Source: CAD feature listing. Evaluate the final solid. Frame: model axes, mm. Face numbers are marked on the shaded views. A direction names the side the tool comes from. Give positions to 0.01 mm unless a question says otherwise; leave off trailing zeros. Loops run counter-clockwise (first coordinate to the right, second up) from the corner with the lowest first, then second, coordinate; pieces in that order, holes last. Notation, with made-up numbers: M 55.5,8.25 L 95.5,8.25 A21 cw 95.5,43.25 Z; hole C 2,88.5 d2. An arc over 180 degrees is marked long. Write item = value, one per line.
from build123d import *

# Parameters (mm, degrees)
BOSS_EXTRUDE2_DEPTH  = 30
BOSS_EXTRUDE3_DEPTH  = 10
BOSS_EXTRUDE4_DEPTH  = 10
BOSS_EXTRUDE7_DEPTH  = 5
CUT_EXTRUDE9_DEPTH   = 10
SKETCH13_R           = 2.5
CUT_EXTRUDE10_DEPTH  = 190
SKETCH14_R           = 15
CUT_EXTRUDE12_DEPTH  = 15
CUT_EXTRUDE13_DEPTH  = 5
BOSS_EXTRUDE8_DEPTH  = 10
SKETCH17_R           = 5
CUT_EXTRUDE15_DEPTH  = 15
CUT_EXTRUDE16_DEPTH  = 5
SKETCH19_W           = 30
SKETCH19_H           = 5
BOSS_EXTRUDE9_DEPTH  = 5
SKETCH20_W           = 30
SKETCH20_H           = 5
BOSS_EXTRUDE10_DEPTH = 5


with BuildPart() as part:
    # Sketch2 → Boss-Extrude2 (new body)
    with BuildSketch(Plane.XY):
        Polygon((-70, 40), (-65, 45), (-5, 45), (0, 40), (0, 0), (-5, -5), (-65, -5), (-70, 0), align=None)
    extrude(amount=BOSS_EXTRUDE2_DEPTH)

    # Sketch4 → Boss-Extrude3 (add)
    with BuildSketch(Plane.XY.offset(30)):
        Polygon((-50, 45), (-45, 50), (-25, 50), (-20, 45), align=None)
    extrude(amount=-BOSS_EXTRUDE3_DEPTH)

    # Sketch5 → Boss-Extrude4 (add)
    with BuildSketch(Plane(origin=(0, 0, 0), x_dir=(-1, 0, 0), z_dir=(0, 0, -1))):
        Polygon((20, 45), (25, 50), (45, 50), (50, 45), align=None)
    extrude(amount=-BOSS_EXTRUDE4_DEPTH)

    # Sketch6 → Boss-Extrude7 (add)
    with BuildSketch(Plane.XY.offset(30)):
        Polygon((-75, 30), (5, 30), (5, 35), (-10, 35), (-10, 45), (-60, 45), (-60, 35), (-75, 35), align=None)
        Polygon((-75, 10), (5, 10), (5, 5), (-10, 5), (-10, -5), (-60, -5), (-60, 5), (-75, 5), align=None)
    extrude(amount=BOSS_EXTRUDE7_DEPTH)

    # Sketch12 → Cut-Extrude9 (cut)
    with BuildSketch(Plane.XY.offset(30)):
        with BuildLine():
            Line((-70, 25), (-60, 25))
            ThreePointArc((-60, 25), (-55, 20), (-60, 15))
            Line((-60, 15), (-70, 15))
            Line((-70, 15), (-70, 25))
        make_face()
        with BuildLine():
            Line((0, 15), (-10, 15))
            ThreePointArc((-10, 15), (-15, 20), (-10, 25))
            Line((-10, 25), (0, 25))
            Line((0, 25), (0, 15))
        make_face()
    extrude(amount=-CUT_EXTRUDE9_DEPTH, mode=Mode.SUBTRACT)

    # Sketch13 → Cut-Extrude10 (cut)
    with BuildSketch(Plane.XY.offset(20)):
        with Locations((-60, 20)):
            Circle(SKETCH13_R)
        with Locations((-10, 20)):
            Circle(SKETCH13_R)
    extrude(amount=-CUT_EXTRUDE10_DEPTH, mode=Mode.SUBTRACT)

    # Sketch14 → Cut-Extrude12 (cut)
    with BuildSketch(Plane.XY.offset(30)):
        with Locations((-35, 20)):
            Circle(SKETCH14_R)
    extrude(amount=-CUT_EXTRUDE12_DEPTH, mode=Mode.SUBTRACT)

    # Sketch15 → Cut-Extrude13 (cut)
    with BuildSketch(Plane.XY.offset(35)):
        with BuildLine():
            Line((-46.180339887, 10), (-23.819660113, 10))
            ThreePointArc((-23.819660113, 10), (-35, 5), (-46.180339887, 10))
        make_face()
        with BuildLine():
            Line((-46.180339887, 30), (-23.819660113, 30))
            ThreePointArc((-23.819660113, 30), (-35, 35), (-46.180339887, 30))
        make_face()
    extrude(amount=-CUT_EXTRUDE13_DEPTH, mode=Mode.SUBTRACT)

    # Sketch16 → Boss-Extrude8 (add)
    with BuildSketch(Plane.XY.offset(35)):
        with BuildLine():
            ThreePointArc((-17.679491924, 10), (-35, 0), (-52.320508076, 10))
            Line((-52.320508076, 10), (-46.180339887, 10))
            ThreePointArc((-46.180339887, 10), (-35, 5), (-23.819660113, 10))
            Line((-23.819660113, 10), (-17.679491924, 10))
        make_face()
        with BuildLine():
            Line((-52.320508076, 30), (-46.180339887, 30))
            ThreePointArc((-46.180339887, 30), (-35, 35), (-23.819660113, 30))
            Line((-23.819660113, 30), (-17.679491924, 30))
            ThreePointArc((-17.679491924, 30), (-35, 40), (-52.320508076, 30))
        make_face()
    extrude(amount=BOSS_EXTRUDE8_DEPTH)

    # Sketch17 → Cut-Extrude15 (cut)
    with BuildSketch(Plane.XY.offset(15)):
        with Locations((-35, 20)):
            Circle(SKETCH17_R)
    extrude(amount=-CUT_EXTRUDE15_DEPTH, mode=Mode.SUBTRACT)

    # Sketch18 → Cut-Extrude16 (cut)
    with BuildSketch(Plane(origin=(0, 0, 0), x_dir=(-1, 0, 0), z_dir=(0, 0, -1))):
        Polygon((5, -5), (10, -5), (10, 5), (0, 5), (0, 0), align=None)
        Polygon((0, 40), (0, 35), (10, 35), (10, 45), (5, 45), align=None)
        Polygon((60, 45), (60, 35), (70, 35), (70, 40), (65, 45), align=None)
        Polygon((70, 0), (70, 5), (60, 5), (60, -5), (65, -5), align=None)
    extrude(amount=-CUT_EXTRUDE16_DEPTH, mode=Mode.SUBTRACT)

    # Sketch19 → Boss-Extrude9 (add)
    with BuildSketch(Plane.ZY.offset(70)):
        with Locations((15, 32.5)):
            Rectangle(SKETCH19_W, SKETCH19_H)
        with Locations((15, 7.5)):
            Rectangle(SKETCH19_W, SKETCH19_H)
    extrude(amount=BOSS_EXTRUDE9_DEPTH)

    # Sketch20 → Boss-Extrude10 (add)
    with BuildSketch(Plane(origin=(0, 0, 0), x_dir=(0, 0, -1), z_dir=(1, 0, 0))):
        with Locations((-15, 32.5)):
            Rectangle(SKETCH20_W, SKETCH20_H)
        with Locations((-15, 7.5)):
            Rectangle(SKETCH20_W, SKETCH20_H)
    extrude(amount=BOSS_EXTRUDE10_DEPTH)


solid = part.part
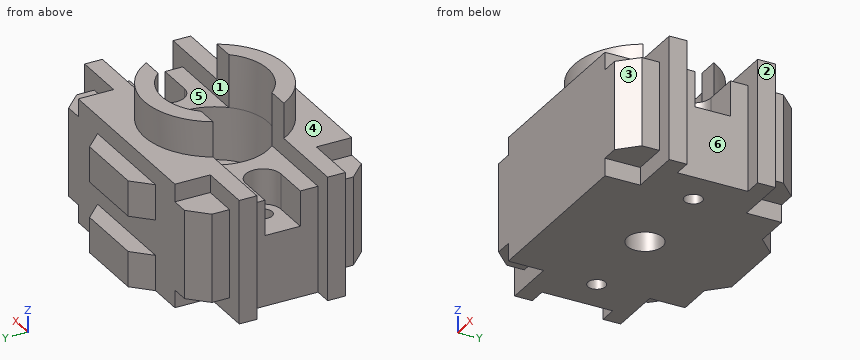
1. First-contact query: pin 1 Ø11 at (x, y) = (-7, 22.5) entering from +Z; pin 2 Ø8 at (x, y) = (-65, -2) entering from -Z; pin 3 Ø6 at (x, z) = (-24.5, 15) entering from +Y; pin 4 Ø9 at (x, y) = (-35, 20) entering from +Z. Flat tips, straight axial feed; report the tip coordinate or a pass-through.
Derived:
pin_1 = 30
pin_2 = 5
pin_3 = 45
pin_4 = through
2. Reachability of the marked faces 4, 5 and 6 from +Z, -Z, +X, -X, +Y, -Y: full face, straight path, thin tool, end or side. Return the list, or none.
Derived:
face_4 = +Z, -Y
face_5 = +Z, +X, -X
face_6 = +Z, -Z, +X
3. Material intervals for probe 1 along Y at (x, z) = (2.5, 29.5); probe 2 along Y at (x, z) = (-62.5, 24); probe 3 along Z at (x, y) = (-69, 8.5), sorted ascending. Write a range as from..to.
Derived:
probe_1 = 5..10, 30..35
probe_2 = -5..15, 25..45
probe_3 = 0..35
4. Cut plane A-A, the plane z = 40.5. Return the cut outline in (x, y), then the cut area to 3 significant figures.
Derived:
outline = M -52.32,10 A20 ccw -17.68,10 L -23.82,10 A15 cw -46.18,10 Z; M -52.32,30 L -46.18,30 A15 cw -23.82,30 L -17.68,30 A20 ccw Z
area = 336 mm²
5. Cut plane C-C, the plane y = 20. Return the cut outline in (x, z), then the cut area to 3 significant figures.
Derived:
outline = M -70,0 L -62.5,0 L -62.5,20 L -70,20 Z; M -57.5,0 L -40,0 L -40,15 L -50,15 L -50,30 L -55,30 L -55,20 L -57.5,20 Z; M -30,0 L -12.5,0 L -12.5,20 L -15,20 L -15,30 L -20,30 L -20,15 L -30,15 Z; M -7.5,0 L 0,0 L 0,20 L -7.5,20 Z
area = 1,000 mm²
6. Cut plane B-B, the plane x = -19. Return the cut outline in (y, z), then the cut area to 3 significant figures.
Derived:
outline = M -5,0 L 45,0 L 45,35 L 32,35 L 32,45 L 30,45 L 30,30 L 10,30 L 10,45 L 8,45 L 8,35 L -5,35 Z
area = 1,690 mm²
7. Pull-direction query (Y, two-part tool) for the marked faces 1, 2 and 3; classes: +Y half, -Y half, draft (parallel to the pull), parting line (faces both ways), or undercut.
Derived:
face_1 = undercut
face_2 = draft
face_3 = -Y half
8. Cut plane D-D, the plane x = -35. Return the cut outline in (y, z), then the cut area to 3 significant figures.
Derived:
outline = M -5,0 L 15,0 L 15,15 L 5,15 L 5,45 L 0,45 L 0,35 L -5,35 Z; M 25,0 L 50,0 L 50,10 L 45,10 L 45,20 L 50,20 L 50,30 L 45,30 L 45,35 L 40,35 L 40,45 L 35,45 L 35,15 L 25,15 Z
area = 1,200 mm²
